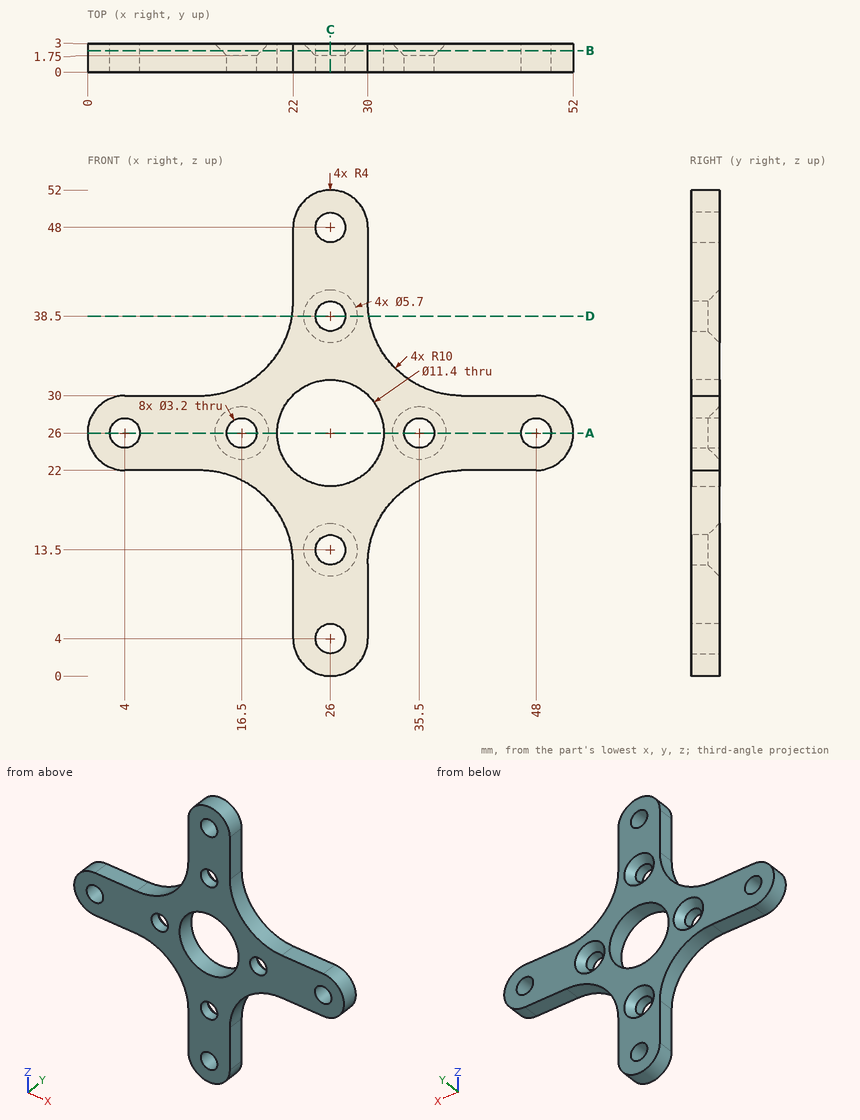
The figure shows three views and two pictorial views of one solid part (mm, origin at its lowest corner). Answer the questions. Coordinates: 2 decimals unless noted, no trailing zeros. Order: outer loops, then holes, each group sorted by start corner. A loop starts at its lowest first (then second) coordinate and runs counter-clockwise, first axis right, second up.
Q1. A cutting plane is placed at C-C, the plane x = 26. Write down the section's boundary in (y, z).
Q2. A cutting plane is placed at B-B, the plane y = 2.3. State how many separate pieces and enclosed holes the cut face has, and give its area (3 significant figures).
Q3. A cutting plane is placed at D-D, the plane z = 38.5. Write down the section's boundary in (x, y).
Q4. Consider line 1 (X direction, y = 0.4, z = 26); line 2 (X direction, y = 2.25, z = 45.5); line 3 (Z direction, x = 15.5, y = 2.35). Determine where each line is inside the solid, lowest interval first.
Q5. Given P1, Ø6, axis at x = 23.5, z = 28, coming from the +Y side; P2, Ø0.9, axis at x = 10, y = 2, coming from the -Z side; P3, Ø3, axis at x = 26, z = 48, coming from the -Y side; P4, Ø3.5, axis at x = 26, z = 13.5, coming from the +Y side, each flat-ended and moving along its own axis, determine where each tip first touches the part or whether it passes through.
Q6. A cutting plane is placed at A-A, the plane z = 26. Write down the section's boundary in (x, y), and give its area (3 significant figures).
Answers follow:
1. outline: (0, 0) - (3, 0) - (3, 2.4) - (0, 2.4) - close; (0, 5.6) - (3, 5.6) - (3, 10.65) - (1.75, 11.9) - (0, 11.9) - close; (0, 15.1) - (1.75, 15.1) - (3, 16.35) - (3, 20.3) - (0, 20.3) - close; (0, 31.7) - (3, 31.7) - (3, 35.65) - (1.75, 36.9) - (0, 36.9) - close; (0, 40.1) - (1.75, 40.1) - (3, 41.35) - (3, 46.4) - (0, 46.4) - close; (0, 49.6) - (3, 49.6) - (3, 52) - (0, 52) - close
2. separate pieces: 1
2. enclosed holes: 9
2. area: 634 mm2
3. outline: (21.89, 0) - (24.4, 0) - (24.4, 1.75) - (23.15, 3) - (21.89, 3) - close; (27.6, 0) - (30.11, 0) - (30.11, 3) - (28.85, 3) - (27.6, 1.75) - close
4. line 1: x = 0 to 2.4, 5.6 to 14.9, 18.1 to 20.3, 31.7 to 33.9, 37.1 to 46.4, 49.6 to 52
4. line 2: x = 22 to 30
4. line 3: z = 21.37 to 24.04, 27.96 to 30.63
5. P1: stops at y = 3
5. P2: stops at z = 22
5. P3: passes through
5. P4: stops at y = 1.9
6. outline: (0, 0) - (2.4, 0) - (2.4, 3) - (0, 3) - close; (5.6, 0) - (14.9, 0) - (14.9, 1.75) - (13.65, 3) - (5.6, 3) - close; (18.1, 0) - (20.3, 0) - (20.3, 3) - (19.35, 3) - (18.1, 1.75) - close; (31.7, 0) - (33.9, 0) - (33.9, 1.75) - (32.65, 3) - (31.7, 3) - close; (37.1, 0) - (46.4, 0) - (46.4, 3) - (38.35, 3) - (37.1, 1.75) - close; (49.6, 0) - (52, 0) - (52, 3) - (49.6, 3) - close
6. area: 80.3 mm2
